Verification items for the finished model (mm, model axes). A direction names the side the tool comes from. Round coordinates to 2 decimals unless told otherwise and drop trailing zeros. Loops run counter-clockwise (first coordinate to the right, second up) from the corner with the lowest first, then second, coordinate; pieces in that order, holes last. Notation, with made-up numbers: (67.5, -4) -> (108.5, -4) arc R22 ccw to (108.5, 28) -> close; hole circle Ø11 at (56, 66.25). An arc over 180 degrees is marked (long way). Use CSV: the item, a comma, the result in double quotes. Start each with the question number.
```python
from build123d import *

# Parameters (mm, degrees)
BOSS_EXTRUDE1_DEPTH = 12.7
SKETCH2_R           = 1.5875
CUT_EXTRUDE1_DEPTH  = 17.526
SKETCH3_R           = 1.5875
CUT_EXTRUDE2_DEPTH  = 17.526


with BuildPart() as part:
    # Sketch1 → Boss-Extrude1 (new body)
    with BuildSketch(Plane(origin=(0, 0, 0), x_dir=(0, 0, -1), z_dir=(1, 0, 0))):
        with BuildLine():
            Line((0, 0), (49.2125, 0))
            ThreePointArc((49.2125, 0), (50.335032015, 0.464967985), (50.8, 1.5875))
            Line((50.8, 1.5875), (50.8, 50.8))
            Line((50.8, 50.8), (49.2125, 50.8))
            Line((49.2125, 50.8), (49.2125, 4.7625))
            ThreePointArc((49.2125, 4.7625), (48.28256403, 2.51743597), (46.0375, 1.5875))
            Line((46.0375, 1.5875), (0, 1.5875))
            Line((0, 1.5875), (0, 0))
        make_face()
    extrude(amount=BOSS_EXTRUDE1_DEPTH)

    # Sketch2 → Cut-Extrude1 (cut)
    with BuildSketch(Plane.XY.offset(-49.2125)):
        with Locations((6.35, 31.75)):
            Circle(SKETCH2_R)
    extrude(amount=-CUT_EXTRUDE1_DEPTH, mode=Mode.SUBTRACT)

    # Sketch3 → Cut-Extrude2 (cut)
    with BuildSketch(Plane(origin=(0, 1.5875, 0), x_dir=(1, 0, 0), z_dir=(0, 1, 0))):
        with Locations(Location((6.35, 19.05, 0), (0, 0, 270))):
            Circle(SKETCH3_R)
    extrude(amount=-CUT_EXTRUDE2_DEPTH, mode=Mode.SUBTRACT)


solid = part.part
```
Q1. Depth check by flat-ended pin: pin 1 Ø1 at (x, z) = (6, -45) entering from +Y; pin 2 Ø3 at (x, y) = (6.35, 31.75) entering from -Z. Enter the tip coordinate at first touch or a pass-through.
Q2. Thickness scan on L1, parallel to X at y = 0.65, z = -19.05; L2, parallel to X at y = 31, z = -50; L3, parallel to Y at x = 3.25, z = -37.5. Record the ranges inside material, lowest first. Write a range as from..to.
Q3. Tool access check on faces 4 (the face through (6, 1.588, -23)), 5 (the face through (6, 50.8, -50)). Record the directions out of +Z, -Z, +X, -X, +Y, -Y that give a thin tool (end or side, any length) a straight path to the whole face; none if there is none.
Q4. Cross-section at C-C (x = 6.35). State how many separate pieces and enclosed holes the cut face has, and give its area (3 significant figures).
Q5. Cross-section at B-B (z = -19.05). Record the boundary of the cut face in (x, y).
Q6. Release check for a two-part mould opening along Z. For faces 1 (the face through (6.42, 0.805, -20.636)), 2 (the face through (6, 1, 0)), 3 (the face through (6, 0, -24)) record: +Z half, -Z half, draft (parallel to the pull), parting line (faces both ways), or undercut.
Q7. Cross-section at A-A (y = 31.75). Record the boundary of the cut face in (x, z), and give its area (3 significant figures).
Answer list:
1,pin 1,"stops at y = 1.59"
1,pin 2,"passes through"
2,L1,"x = 0..4.76, 7.94..12.7"
2,L2,"x = 0..4.95, 7.75..12.7"
2,L3,"y = 0..1.59"
3,face 4,"+Z, +X, -X, +Y"
3,face 5,"+Z, -Z, +X, -X, +Y"
4,separate pieces,"3"
4,enclosed holes,"0"
4,area,"150 mm2"
5,outline,"(0, 0) -> (4.76, 0) -> (4.76, 1.59) -> (0, 1.59) -> close; (7.94, 0) -> (12.7, 0) -> (12.7, 1.59) -> (7.94, 1.59) -> close"
6,face 1,"undercut"
6,face 2,"+Z half"
6,face 3,"draft"
7,outline,"(0, -50.8) -> (4.76, -50.8) -> (4.76, -49.21) -> (0, -49.21) -> close; (7.94, -50.8) -> (12.7, -50.8) -> (12.7, -49.21) -> (7.94, -49.21) -> close"
7,area,"15.1 mm2"
